For this review, take the finished solid that the model builds, in its own axes (mm). Face numbers are marked on the shaded views. A direction names the side the tool comes from. Coordinates: 2 decimals unless noted, no trailing zeros. Loops run counter-clockwise (first coordinate to the right, second up) from the corner with the lowest first, then second, coordinate; pieces in that order, holes last. Notation, with made-up numbers: (53.5, 41.5) -> (64.5, 41.5) arc R30 ccw to (64.5, 73.5) -> close; hole circle Ø9 at (77.5, 87). An arc over 180 degrees is marked (long way). Answer in a Markdown table with one row per item.
from build123d import *

# Parameters (mm, degrees)
SKETCH_1_R      = 7.5
SKETCH_1_R_2    = 1.45
SKETCH_1_W      = 18
SKETCH_1_H      = 18
EXTRUDE_1_DEPTH = 3
FILLET_1_R      = 2


with BuildPart() as part:
    # 草图1 → 凸台-拉伸1 (new body)
    with BuildSketch(Plane.XY):
        with BuildLine():
            Line((-15, 35), (-15, -5))
            Line((-15, -5), (15, -5))
            Line((15, -5), (15, 35))
            ThreePointArc((15, 35), (0, 50), (-15, 35))
        make_face()
        with Locations((0, 35)):
            Circle(SKETCH_1_R, mode=Mode.SUBTRACT)
        with Locations((-10, 0)):
            Circle(SKETCH_1_R_2, mode=Mode.SUBTRACT)
        with Locations((10, 0)):
            Circle(SKETCH_1_R_2, mode=Mode.SUBTRACT)
        with Locations((0, 14)):
            Rectangle(SKETCH_1_W, SKETCH_1_H, mode=Mode.SUBTRACT)
    extrude(amount=EXTRUDE_1_DEPTH)

    # 圆角1
    fillet_1_edges = [part.edges().sort_by_distance(p)[0] for p in [
        (9, 5, 1.5),
        (9, 23, 1.5),
        (-9, 23, 1.5),
        (-9, 5, 1.5),
        (15, -5, 1.5),
        (-15, -5, 1.5),
    ]]
    fillet(fillet_1_edges, radius=FILLET_1_R)


solid = part.part
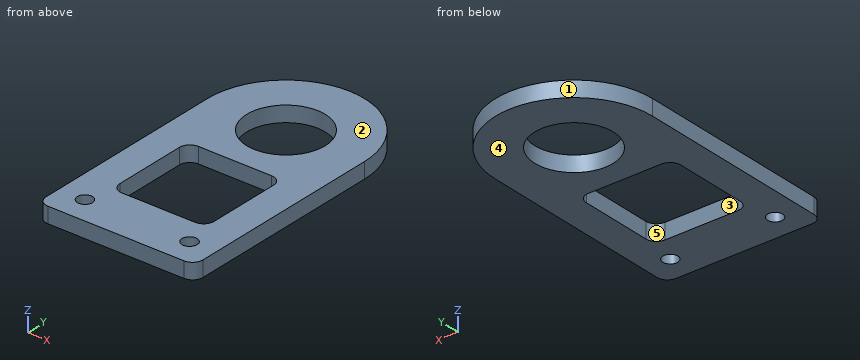
Item 1: For L1, parallel to Y at x = 6.5, z = 2.4; L2, parallel to Y at x = 0, z = 1.6; L3, parallel to X at y = 20, z = 1.2, list the stretches that pass through material, from the lowest coordinate up.
Worked answers:
| item | result |
|---|---|
| L1 | -5 to 5, 23 to 31.26, 38.74 to 48.52 |
| L2 | -5 to 5, 23 to 27.5, 42.5 to 50 |
| L3 | -15 to -9, 9 to 15 |
Item 2: Take a section at B-B, the plane y = 17. State the section outline as (x, z) points, and give its area (3 significant figures).
Worked answers:
| item | result |
|---|---|
| outline | (-15, 0) -> (-9, 0) -> (-9, 3) -> (-15, 3) -> close; (9, 0) -> (15, 0) -> (15, 3) -> (9, 3) -> close |
| area | 36.0 mm² |
Item 3: Take a section at A-A, the plane x = 0. State the section outline as (y, z) points, and give its area (3 significant figures).
Worked answers:
| item | result |
|---|---|
| outline | (-5, 0) -> (5, 0) -> (5, 3) -> (-5, 3) -> close; (23, 0) -> (27.5, 0) -> (27.5, 3) -> (23, 3) -> close; (42.5, 0) -> (50, 0) -> (50, 3) -> (42.5, 3) -> close |
| area | 66.0 mm² |
Item 4: Take a section at C-C, the plane z = 1.7. State the section outline as (x, y) points, and give its area (3 significant figures).
Worked answers:
| item | result |
|---|---|
| outline | (-15, -3) arc R2 ccw to (-13, -5) -> (13, -5) arc R2 ccw to (15, -3) -> (15, 35) arc R15 ccw to (-15, 35) -> close; hole circle Ø2.9 at (-10, 0); hole (-9, 7) arc R2 ccw to (-7, 5) -> (7, 5) arc R2 ccw to (9, 7) -> (9, 21) arc R2 ccw to (7, 23) -> (-7, 23) arc R2 ccw to (-9, 21) -> close; hole circle Ø15 at (0, 35); hole circle Ø2.9 at (10, 0) |
| area | 1,040 mm² |
Item 5: Take a section at D-D, the plane x = 10. State the section outline as (y, z) points, and give its area (3 significant figures).
Worked answers:
| item | result |
|---|---|
| outline | (-5, 0) -> (-1.45, 0) -> (-1.45, 3) -> (-5, 3) -> close; (1.45, 0) -> (46.18, 0) -> (46.18, 3) -> (1.45, 3) -> close |
| area | 145 mm² |
Item 6: Insertion check: pin 1 (0.9 mm diameter, centred on x = 2, z = 1.5, fed in from +Y); pin 2 (2 mm diameter, centred on x = 0, y = 20.5, fed in from +Z); pin 3 (1.5 mm diameter, centred on y = 37.5, z = 2, fed in from -X). Each pin has a flat end and moves straight along its axis. Give the tip position at first contact, or say it passes through.
Worked answers:
| item | result |
|---|---|
| pin 1 | y = 49.92 |
| pin 2 | through |
| pin 3 | x = -14.9 |
Item 7: The part is to be moulded in two halves that separate along X. For the marked faces 1, 2 and 3, say which applies: +X half, -X half, draft (parallel to the pull), parting line (faces both ways), or undercut.
Worked answers:
| item | result |
|---|---|
| face 1 | parting line |
| face 2 | draft |
| face 3 | undercut |
Item 8: For the marked faces 4 and 5, list the 3-axis set-ups (+Z, -Z, +X, -X, +Y, -Y) from which the entire face can be reached by the end or side of a thin tool; tool diameter is ignored.
Worked answers:
| item | result |
|---|---|
| face 4 | -Z, +X, -X, +Y, -Y |
| face 5 | +Z, -Z |
